from build123d import *

# Parameters (mm, degrees)
SKETCH2_R          = 3
CUT_EXTRUDE1_DEPTH = 23.5


with BuildPart() as part:
    # Sketch1 → Revolve1 (revolve)
    with BuildSketch(Plane.XY, mode=Mode.PRIVATE) as revolve1_sk:
        Polygon((-73.063744965, 4.5), (0, 4.5), (0, 34.5), (-2.67228246, 34.5), (-5.556499615, 24.5), (-11.556499615, 24.5), (-15.990247298, 34.5), (-18.237315581, 34.5), (-18.237315581, 27.5), (-19.962759183, 27.5), (-22.377341153, 18.5), (-28.377341153, 18.5), (-30.883350481, 27.5), (-34.250598113, 27.5), (-34.250598113, 22.5), (-35.976041715, 22.5), (-38.65891057, 12.5), (-44.65891057, 12.5), (-47.443365379, 22.5), (-50.057907164, 22.5), (-50.057907164, 15), (-51.783350766, 15), (-53.393072079, 9), (-59.393072079, 9), (-61.063744965, 15), (-73.063744965, 15), align=None)
    revolve(revolve1_sk.sketch.rotate(Axis((0, 0, 0), (-1, 0, 0)), 90), axis=Axis((0, 0, 0), (-1, 0, 0)))

    # Sketch2 → Cut-Extrude1 (cut, symmetric)
    with BuildSketch(Plane(origin=(0, 0, 0), x_dir=(1, 0, 0), z_dir=(0, 1, 0))):
        with Locations(Location((-67.063744965, 0, 0), (0, 0, 270))):
            Circle(SKETCH2_R)
    extrude(amount=CUT_EXTRUDE1_DEPTH, both=True, mode=Mode.SUBTRACT)


solid = part.part
Could you check a few things on this model? Use its own coordinates, in mm. A direction names the side the tool comes from. Give positions to 0.01 mm unless a question says otherwise; leave off trailing zeros. Order: outer loops, then holes, each group sorted by start corner. A loop starts at its lowest first (then second) coordinate and runs counter-clockwise, first axis right, second up.
Item 1: If we section it at A-A, the plane x = -55: Write out the boundary of the cut face in (y, z), plus the area to 3 significant figures.
Item 2: I'm going to push flat-ended pins straight in: pin 1 (4 mm diameter, centred on x = -17.5, y = -22.5, fed in from -Z); pin 2 (1.5 mm diameter, centred on y = -21.5, z = -16.5, fed in from -X); pin 3 (7 mm diameter, centred on x = -67.06, z = 0, fed in from +Y). Where does each tip first touch, or does it pass through?
Item 3: For faces 4 (the face through (-5.416, 24.391, 5.416)), 5 (the face through (-32.591, 24.397, -12.69)), 6 (the face through (-1.355, -1.517, 34.467)), which set-ups out of +Z, -Z, +X, -X, +Y, -Y let a thin tool reach every point of the face, with its end or its side?
Item 4: If we section it at B-B, the plane z = 0: Count the separate pieces of the cut face and the enclosed holes in it, plus the area to 3 significant figures.
Item 5: If we mould it in two halves opening along X, with no side actions, what happens to faces 1 (the face through (-34.251, 0, 23)), 2 (the face through (-50.93, -12.65, -8.06)), 3 (the face through (-25.42, 16.41, -8.54))? For each: pulls with the +X half, pulls with the -X half, needs draft (parallel to the pull), parting line crosses it, or undercut.
Item 6: I need wall thicknesses on line 1 (X direction, y = 6, z = 0); line 2 (X direction, y = 9, z = -23); line 3 (X direction, y = 6, z = -31). Which ranges of each line are inside material? Lowest first, please.
Values:
1. outline: circle Ø18 at (0, 0); hole circle Ø9 at (0, 0)
1. area: 191 mm2
2. pin 1: stops at z = -27.75
2. pin 2: stops at x = -34.25
2. pin 3: stops at y = 15
3. face 4: none
3. face 5: -X
3. face 6: +X, -X
4. separate pieces: 4
4. enclosed holes: 0
4. area: 2,150 mm2
5. face 1: pulls with the -X half
5. face 2: needs draft
5. face 3: undercut
6. line 1: x = -73.06 to -70.06, -64.06 to 0
6. line 2: x = -34.25 to -30.1, -20.71 to -11.64, -5.5 to 0
6. line 3: x = -18.24 to -14.69, -3.52 to 0
